from build123d import *

# Parameters (mm, degrees)
F0_R     = 9.525
F1_DEPTH = 19.05
F0_R_2   = 12.7
F2_DEPTH = 38.1
F3_DEPTH = 50.8


with BuildPart() as f1:
    # F0 (on Top) → F1 (new body)
    with BuildSketch(Plane.XY):
        with BuildLine():
            Line((20.6375, -35.745199), (58.7375, -13.748153))
            ThreePointArc((58.7375, -13.748153), (66.675, 0), (58.7375, 13.748153))
            Line((58.7375, 13.748153), (20.6375, 35.745199))
            ThreePointArc((20.6375, 35.745199), (0, 41.275), (-20.6375, 35.745199))
            Line((-20.6375, 35.745199), (-58.7375, 13.748153))
            ThreePointArc((-58.7375, 13.748153), (-66.675, 0), (-58.7375, -13.748153))
            Line((-58.7375, -13.748153), (-20.6375, -35.745199))
            ThreePointArc((-20.6375, -35.745199), (0, -41.275), (20.6375, -35.745199))
        make_face()
        with Locations((-50.8, 0)):
            Circle(F0_R, mode=Mode.SUBTRACT)
        with BuildLine():
            ThreePointArc((6.35, 34.342876), (24.695704, 24.695704), (34.342876, 6.35))
            ThreePointArc((34.342876, 6.35), (34.779164, 3.188313), (34.925, 0))
            ThreePointArc((34.925, 0), (34.779164, -3.188313), (34.342876, -6.35))
            ThreePointArc((34.342876, -6.35), (24.695704, -24.695704), (6.35, -34.342876))
            ThreePointArc((6.35, -34.342876), (0, -34.925), (-6.35, -34.342876))
            ThreePointArc((-6.35, -34.342876), (-24.695704, -24.695704), (-34.342876, -6.35))
            ThreePointArc((-34.342876, -6.35), (-34.925, 0), (-34.342876, 6.35))
            ThreePointArc((-34.342876, 6.35), (-24.695704, 24.695704), (-6.35, 34.342876))
            ThreePointArc((-6.35, 34.342876), (0, 34.925), (6.35, 34.342876))
        make_face(mode=Mode.SUBTRACT)
        with Locations((50.8, 0)):
            Circle(F0_R, mode=Mode.SUBTRACT)
    extrude(amount=F1_DEPTH)

    # F0 (on Top) → F2 (join)
    with BuildSketch(Plane.XY):
        with BuildLine():
            Line((6.35, -34.342876), (6.35, -24.593444))
            ThreePointArc((6.35, -24.593444), (0, -25.4), (-6.35, -24.593444))
            Line((-6.35, -24.593444), (-6.35, -34.342876))
            ThreePointArc((-6.35, -34.342876), (0, -34.925), (6.35, -34.342876))
        make_face()
        with BuildLine():
            Line((-6.35, -34.342876), (-6.35, -24.593444))
            ThreePointArc((-6.35, -24.593444), (-17.960512, -17.960512), (-24.593444, -6.35))
            Line((-24.593444, -6.35), (-34.342876, -6.35))
            ThreePointArc((-34.342876, -6.35), (-24.695704, -24.695704), (-6.35, -34.342876))
        make_face()
        with BuildLine():
            Line((34.342876, -6.35), (24.593444, -6.35))
            ThreePointArc((24.593444, -6.35), (17.960512, -17.960512), (6.35, -24.593444))
            Line((6.35, -24.593444), (6.35, -34.342876))
            ThreePointArc((6.35, -34.342876), (24.695704, -24.695704), (34.342876, -6.35))
        make_face()
        with BuildLine():
            ThreePointArc((24.593444, -6.35), (25.197554, -3.200509), (25.4, 0))
            ThreePointArc((25.4, 0), (25.197554, 3.200509), (24.593444, 6.35))
            ThreePointArc((24.593444, 6.35), (17.960512, 17.960512), (6.35, 24.593444))
            ThreePointArc((6.35, 24.593444), (0, 25.4), (-6.35, 24.593444))
            ThreePointArc((-6.35, 24.593444), (-17.960512, 17.960512), (-24.593444, 6.35))
            ThreePointArc((-24.593444, 6.35), (-25.4, 0), (-24.593444, -6.35))
            ThreePointArc((-24.593444, -6.35), (-17.960512, -17.960512), (-6.35, -24.593444))
            ThreePointArc((-6.35, -24.593444), (0, -25.4), (6.35, -24.593444))
            ThreePointArc((6.35, -24.593444), (17.960512, -17.960512), (24.593444, -6.35))
        make_face()
        Circle(F0_R_2, mode=Mode.SUBTRACT)
        with BuildLine():
            ThreePointArc((24.593444, 6.35), (25.197554, 3.200509), (25.4, 0))
            ThreePointArc((25.4, 0), (25.197554, -3.200509), (24.593444, -6.35))
            Line((24.593444, -6.35), (34.342876, -6.35))
            ThreePointArc((34.342876, -6.35), (34.779164, -3.188313), (34.925, 0))
            ThreePointArc((34.925, 0), (34.779164, 3.188313), (34.342876, 6.35))
            Line((34.342876, 6.35), (24.593444, 6.35))
        make_face()
        with BuildLine():
            ThreePointArc((6.35, 24.593444), (17.960512, 17.960512), (24.593444, 6.35))
            Line((24.593444, 6.35), (34.342876, 6.35))
            ThreePointArc((34.342876, 6.35), (24.695704, 24.695704), (6.35, 34.342876))
            Line((6.35, 34.342876), (6.35, 24.593444))
        make_face()
        with BuildLine():
            ThreePointArc((-24.593444, -6.35), (-25.4, 0), (-24.593444, 6.35))
            Line((-24.593444, 6.35), (-34.342876, 6.35))
            ThreePointArc((-34.342876, 6.35), (-34.925, 0), (-34.342876, -6.35))
            Line((-34.342876, -6.35), (-24.593444, -6.35))
        make_face()
        with BuildLine():
            ThreePointArc((-24.593444, 6.35), (-17.960512, 17.960512), (-6.35, 24.593444))
            Line((-6.35, 24.593444), (-6.35, 34.342876))
            ThreePointArc((-6.35, 34.342876), (-24.695704, 24.695704), (-34.342876, 6.35))
            Line((-34.342876, 6.35), (-24.593444, 6.35))
        make_face()
        with BuildLine():
            ThreePointArc((-6.35, 24.593444), (0, 25.4), (6.35, 24.593444))
            Line((6.35, 24.593444), (6.35, 34.342876))
            ThreePointArc((6.35, 34.342876), (0, 34.925), (-6.35, 34.342876))
            Line((-6.35, 34.342876), (-6.35, 24.593444))
        make_face()
    extrude(amount=F2_DEPTH)

    # F0 (on Top) → F3 (join)
    with BuildSketch(Plane.XY):
        with BuildLine():
            ThreePointArc((6.35, 24.593444), (17.960512, 17.960512), (24.593444, 6.35))
            Line((24.593444, 6.35), (34.342876, 6.35))
            ThreePointArc((34.342876, 6.35), (24.695704, 24.695704), (6.35, 34.342876))
            Line((6.35, 34.342876), (6.35, 24.593444))
        make_face()
        with BuildLine():
            Line((34.342876, -6.35), (24.593444, -6.35))
            ThreePointArc((24.593444, -6.35), (17.960512, -17.960512), (6.35, -24.593444))
            Line((6.35, -24.593444), (6.35, -34.342876))
            ThreePointArc((6.35, -34.342876), (24.695704, -24.695704), (34.342876, -6.35))
        make_face()
        with BuildLine():
            Line((-6.35, -34.342876), (-6.35, -24.593444))
            ThreePointArc((-6.35, -24.593444), (-17.960512, -17.960512), (-24.593444, -6.35))
            Line((-24.593444, -6.35), (-34.342876, -6.35))
            ThreePointArc((-34.342876, -6.35), (-24.695704, -24.695704), (-6.35, -34.342876))
        make_face()
        with BuildLine():
            ThreePointArc((-24.593444, 6.35), (-17.960512, 17.960512), (-6.35, 24.593444))
            Line((-6.35, 24.593444), (-6.35, 34.342876))
            ThreePointArc((-6.35, 34.342876), (-24.695704, 24.695704), (-34.342876, 6.35))
            Line((-34.342876, 6.35), (-24.593444, 6.35))
        make_face()
    extrude(amount=F3_DEPTH)


solid = f1.part
Source: CAD feature listing. Evaluate the final solid. Frame: model axes, mm. A direction names the side the tool comes from. Round coordinates to 2 decimals unless told otherwise and drop trailing zeros. Write each loop counter-clockwise with the first axis right and the second up, starting at its lowest first coordinate (ties: lowest second). Pieces come first, ordered by that corner, then holes. Notation, with made-up numbers: M 29.5,30.25 L 64.5,30.25 A20 cw 64.5,37.25 Z; hole C 53,-39 d6. An arc over 180 degrees is marked long. One line per item, written item: value. Start each with the question number.
Item 1: Section query C-C (z = 15). State how many separate pieces and enclosed holes the cut face has, plus the area to 3 significant figures.
Item 2: Section query B-B (z = 46.5). Return the cut outline in (x, y) (3 decimals).
Item 3: Pin query (flat end, axial travel): pin 1 (8 mm diameter, centred on y = -28, z = 43, fed in from +X); pin 2 (2 mm diameter, centred on x = 12, z = 44.5, fed in from +Y); pin 3 (1 mm diameter, centred on x = 18, z = 29.5, fed in from +Y); pin 4 (10 mm diameter, centred on x = 39, y = 12, fed in from -Z). Return the tip coordinate at first contact, or that it passes through.
Item 4: Section query D-D (z = 22.5). Return the cut outline in (x, y) (3 decimals), plus the area to 3 significant figures.
Item 5: Ray query, L1, parallel to Y at x = 0, z = 28 (3 decimals); L2, parallel to X at y = 19.5, z = 42.5; L3, parallel to Y at x = 11.5, z = 21.5. Return the intervals inside material, ascending. Write a range as from..to.
Item 6: Set-up query: faces 4 (the flat face through (20, -20, 50.8)), 5 (the flat face through (29, 6.35, 44)), 6 (the flat face through (6.35, 30, 44)), 7 (the cylindrical face through (-17.83, -18.09, 44.36)), 8 (the flat face through (-39.42, 24.9, 9.39)). Return all of +Z, -Z, +X, -X, +Y, -Y with unobstructed straight access to the full face (end or side cutting, diameter ignored); none if empty.
Item 7: Section query A-A (x = 0). Return the cut outline in (y, z) (3 decimals).
Item 8: Mould query, pull axis X, two halves, no side actions, for faces 1 (the flat face through (-39.954, -24.593, 9.392)), 2 (the cylindrical face through (59.6, -3.65, 9.39)), 3 (the flat face through (30, -6.35, 44)). Classes: pulls with the +X half, pulls with the -X half, needs draft (parallel to the pull), parting line crosses it, or undercut.
Result set:
1. separate pieces: 1
1. enclosed holes: 3
1. area: 6,260 mm²
2. outline: M -34.343,-6.35 A34.925 ccw -6.35,-34.343 L -6.35,-24.593 A25.4 cw -24.593,-6.35 Z; M -34.343,6.35 L -24.593,6.35 A25.4 cw -6.35,24.593 L -6.35,34.343 A34.925 ccw Z; M 6.35,-34.343 A34.925 ccw 34.343,-6.35 L 24.593,-6.35 A25.4 cw 6.35,-24.593 Z; M 6.35,24.593 A25.4 cw 24.593,6.35 L 34.343,6.35 A34.925 ccw 6.35,34.343 Z
3. pin 1: stops at x = 25.37
3. pin 2: stops at y = 33.15
3. pin 3: stops at y = 30.22
3. pin 4: stops at z = 0
4. outline: M -34.343,-6.35 A34.925 ccw -6.35,-34.343 A34.925 ccw 6.35,-34.343 A34.925 ccw 34.343,-6.35 A34.925 ccw 34.925,0 A34.925 ccw 34.343,6.35 A34.925 ccw 6.35,34.343 A34.925 ccw -6.35,34.343 A34.925 ccw -34.343,6.35 A34.925 ccw Z; hole C 0,0 d25.4
4. area: 3,330 mm²
5. L1: y = -34.925..-12.7, 12.7..34.925
5. L2: x = -28.97..-16.28, 16.28..28.97
5. L3: y = -32.98..-5.39, 5.39..32.98
6. face 4: +Z, +X, -X, +Y, -Y
6. face 5: +Z, +X, -X
6. face 6: +Z, +Y, -Y
6. face 7: +Z
6. face 8: +Z, -Z, -X, +Y
7. outline: M -41.275,0 L -12.7,0 L -12.7,38.1 L -34.925,38.1 L -34.925,19.05 L -41.275,19.05 Z; M 12.7,0 L 41.275,0 L 41.275,19.05 L 34.925,19.05 L 34.925,38.1 L 12.7,38.1 Z
8. face 1: pulls with the -X half
8. face 2: undercut
8. face 3: needs draft
